Geometry check sheet. Reference: the model listing, model coordinates, mm. Face numbers are marked on the shaded views. A direction names the side the tool comes from. Round coordinates to 2 decimals unless told otherwise and drop trailing zeros. Loops run counter-clockwise (first coordinate to the right, second up) from the corner with the lowest first, then second, coordinate; pieces in that order, holes last. Notation, with made-up numbers: (-15.75, 78.25) -> (41.25, 78.25) arc R31 ccw to (41.25, 114.25) -> close; hole circle Ø5 at (-16.5, -30.5). An arc over 180 degrees is marked (long way). Use a Markdown table: item, result. Add a question column.
Q1. Gauge pin test, flat ends, axial feed: P1, Ø6.5, axis at x = -5, z = -3.5, coming from the +Y side; P2, Ø3, axis at x = 0.5, y = 4.5, coming from the -Z side; P3, Ø3, axis at x = -5.68, z = -3.75, coming from the +Y side; P4, Ø5.5, axis at x = 2.15, z = -3.75, coming from the +Y side. Record the tip position at first contact, or that the pin passes through.
Q2. Release check for a two-part mould opening along Z. For the marked faces 1, 2 and 3 record: released by +Z, released by -Z, zero draft, split by the parting line, or undercut.
Q3. Sectioned sample at B-B, the plane z = -6.5. Enter the section's corners in (x, y), then the cut area to 3 significant figures.
Q4. Sectioned sample at C-C, the plane x = -9.5. Enter the section's corners in (y, z), then the cut area to 3 significant figures.
Q5. Sectioned sample at D-D, the plane y = 2.5. Enter the section's corners in (x, z), then the cut area to 3 significant figures.
Q6. Set-up check for the marked faces 4, 5 and 6: record each of +Z, -Z, +X, -X, +Y, -Y from which the full face is reachable in a straight line by a thin tool's end or side.
Q7. Sectioned sample at A-A, the plane x = 2.5. Enter the section's corners in (y, z).
Q8. Material ranges on L1, parallel to Y at x = 2.5, z = 3.75; L2, parallel to X at y = 0.75, z = -3.25; L3, parallel to Z at x = -9, y = 1.5, recorded low to high.
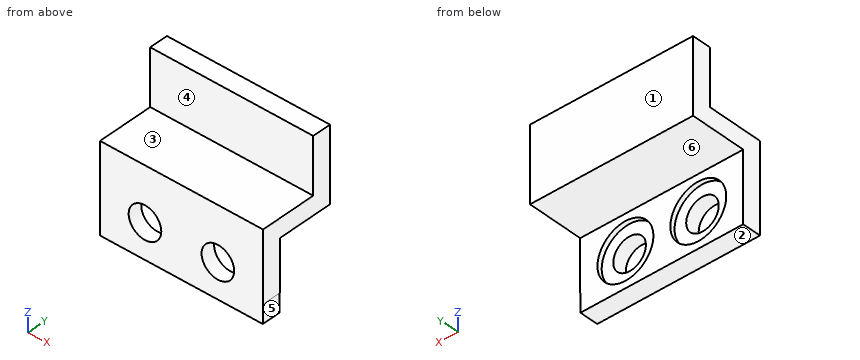
Autodesk Inventor part; units mm, degrees
ref_plane "YZ Plane" through (0, 0, 0) normal (1, 0, 0) x (0, 1, 0)
ref_plane "XZ Plane" through (0, 0, 0) normal (0, 1, 0) x (-1, 0, 0)
ref_plane "XY Plane" through (0, 0, 0) normal (0, 0, 1) x (1, 0, 0)
sketch "Boceto1" plane through (0, 0, 0) normal (0, 1, 0) x (-1, 0, 0)
  line L0 (0, 0) -> (3.5, 0)
  line L1 (3.5, 0) -> (5.5, 0)
  line L2 (0, 0) -> (-2, 0)
  line L3 (-2, -5.5) -> (5.5, -5.5)
  line L4 (-2, 0) -> (-5, 0)
  line L5 (-5, -5.5) -> (-2, -5.5)
  line L6 (5.5, 0) -> (8.5, 0)
  line L7 (8.5, -5.5) -> (5.5, -5.5)
  line L8 (8.5, -5.5) -> (9.5, -5.5)
  line L9 (9.5, 0) -> (8.5, 0)
  line L10 (-5, -5.5) -> (-6, -5.5)
  line L11 (-6, 0) -> (-5, 0)
  line L12 (9.5, -5.5) -> (10.5, -5.5)
  line L13 (10.5, -5.5) -> (10.5, 0)
  line L14 (10.5, 0) -> (9.5, 0)
  line L15 (-6, -5.5) -> (-7, -5.5)
  line L16 (-7, -5.5) -> (-7, 0)
  line L17 (-7, 0) -> (-6, 0)
  dimension "d30" = 1
  dimension "d37" = 1
  dimension "d38" = 1
extrude "Extrusión3" add sketch "Boceto1" along normal blind 2
sketch "Boceto4" plane through (-8.5, 0, 0) normal (0, 0, 1) x (1, 0, 0)
  line L0 (15.5, 2) -> (-2, 2)
  line L1 (0, 2) -> (13.5, 2)
  line L2 (13.5, 2) -> (13.5, 0)
  line L3 (13.5, 0) -> (0, 0)
  line L4 (0, 0) -> (0, 2)
  point P0 (8.5, 0)
  point P1 (14.5, 2)
  point P2 (-1, 2)
extrude "Extrusión4" add sketch "Boceto4" along normal blind 2
sketch "Boceto5" plane through (0, 2, 0) normal (0, 1, 0) x (1, 0, 0)
  line L0 (-8.5, -2) -> (5, -2)
  line L1 (5, -2) -> (-8.5, -2)
  line L2 (-8.5, -2) -> (-8.5, 0)
  line L3 (-8.5, 0) -> (5, 0)
  line L4 (5, 0) -> (5, -2)
  point P0 (0, 0)
extrude "Extrusión5" add sketch "Boceto5" along normal blind 6
sketch "Boceto6" plane through (-8.5, 0, 2) normal (0, 0, 1) x (1, 0, 0)
  line L0 (0, 0) -> (13.5, 0)
  line L1 (13.5, 0) -> (13.5, 6)
  line L2 (13.5, 6) -> (0, 6)
  line L3 (0, 0) -> (0, 6)
  line L4 (0, 0) -> (13.5, 0)
  line L5 (0, 0) -> (0, 8)
  line L6 (0, 8) -> (13.5, 8)
  line L7 (13.5, 8) -> (13.5, 6)
  line L8 (13.5, 6) -> (0, 6)
  line L9 (0, 6) -> (0, 8)
  point P0 (8.5, 0)
extrude "Extrusión6" add sketch "Boceto6" along normal blind 5 contours L5 L6 L7 L2
sketch "Boceto8" plane through (5, 0, -5.5) normal (0, 0, -1) x (-1, 0, 0)
  line L0 (13.5, 0) -> (13.5, 6)
  line L1 (13.5, 2) -> (0, 2)
  line L2 (13.5, 0) -> (0, 0)
  line L3 (0, 0) -> (0, 2)
  line L4 (0, 2) -> (13.5, 2)
  line L5 (13.5, 2) -> (13.5, 0)
  point P0 (5, 0)
extrude "Extrusión8" add sketch "Boceto8" along normal blind 2
sketch "Boceto11" plane through (5, 0, 2) normal (1, 0, 0) x (0, 0, -1)
  line L0 (-5, 8) -> (2, 8)
  line L1 (2, 8) -> (2, 6)
  line L2 (-5, 6) -> (-5, 8)
  line L3 (0, 0) -> (0, 6)
  line L4 (2, 0) -> (2, 2)
  line L5 (2, 6) -> (2, 0)
  line L6 (2, 0) -> (0, 0)
  line L7 (0, 0) -> (0, 6)
  line L8 (0, 6) -> (-5, 6)
  line L9 (0, 6) -> (-5, 6)
  line L10 (2, 0) -> (0, 0)
  line L11 (0, 0) -> (2, 0)
  line L12 (2, 2) -> (2, 8)
  line L13 (2, 0) -> (2, 8)
  line L14 (2, 8) -> (-5, 8)
  line L15 (2, 8) -> (-5, 8)
  line L16 (-5, 8) -> (-5, 6)
  line L17 (0, 6) -> (0, 0)
extrude "Extrusión11" add sketch "Boceto11" along normal blind 2
sketch "Boceto12" plane through (-8.5, 0, 0) normal (-1, 0, 0) x (0, 0, 1)
  line L0 (0, 8) -> (7, 8)
  line L1 (7, 8) -> (7, 6)
  line L2 (2, 6) -> (7, 6)
  line L3 (7, 6) -> (2, 6)
  line L4 (2, 6) -> (2, 0)
  line L5 (0, 0) -> (2, 0)
  line L6 (2, 0) -> (0, 0)
  line L7 (0, 2) -> (0, 8)
  line L8 (0, 0) -> (0, 8)
  line L9 (0, 8) -> (7, 8)
extrude "Extrusión12" add sketch "Boceto12" along normal blind 2
sketch "Boceto13" plane through (0, 2, 0) normal (0, 1, 0) x (1, 0, 0)
  line L0 (-8.5, 5.5) -> (-10.5, 5.5)
  line L1 (-10.5, 5.5) -> (6.9708, 5.5)
  line L2 (6.9708, 5.5) -> (6.9708, 7.5)
  line L3 (6.9708, 7.5) -> (-10.5, 7.5)
  line L4 (-10.5, 7.5) -> (-10.5, 5.5)
  point P0 (0, 0)
extrude "Extrusión13" add sketch "Boceto13" against normal blind 2
sketch "Boceto14" plane through (0, 2, 0) normal (0, 1, 0) x (1, 0, 0)
  circle A0 centre (2.1471, 3.7519) radius 1.75
  circle A1 centre (-5.6769, 3.7519) radius 1.75
  line L0 (1.1471, 3.7519) -> (2.1471, 3.7519)
  line L1 (-4.6769, 3.7519) -> (-5.6769, 3.7519)
  point P0 (0, 0)
  dimension "d43" = 3.5
  dimension "d44" = 3.5
  dimension "d45" = 1
  dimension "d46" = 1
extrude "Extrusión14" cut sketch "Boceto14" against normal blind 2
sketch "Boceto15" plane through (0, 2, 0) normal (0, 1, 0) x (1, 0, 0)
  circle A0 centre (2.1471, 3.7519) radius 1.75
  circle A1 centre (2.1471, 3.7519) radius 3
  circle A2 centre (-5.6769, 3.7519) radius 1.75
  circle A3 centre (-5.6769, 3.7519) radius 3
  point P0 (0, 0)
  dimension "d49" = 6
  dimension "d50" = 6
extrude "Extrusión15" cut sketch "Boceto15" against normal blind 0.5
sketch "Boceto16" plane through (-8.5, 0, 7) normal (0, 0, 1) x (1, 0, 0)
  line L0 (15.5, 2) -> (15.5, 8)
  line L1 (15.5, 6) -> (-2, 6)
  line L2 (15.5, 8) -> (-2, 8)
  line L3 (-2, 8) -> (-2, 6)
  line L4 (-2, 6) -> (15.5, 6)
  line L5 (15.5, 6) -> (15.5, 8)
  point P0 (8.5, 0)
extrude "Extrusión16" add sketch "Boceto16" along normal blind 1
properties part number "Pantalla - encaix slider"
Values:
| question | item | result |
|---|---|---|
| 1 | P1 | y = 2 |
| 1 | P2 | z = 0 |
| 1 | P3 | through |
| 1 | P4 | y = 1.5 |
| 2 | face 1 | zero draft |
| 2 | face 2 | released by -Z |
| 2 | face 3 | released by +Z |
| 3 | outline | (-10.5, 0) -> (6.97, 0) -> (6.97, 2) -> (3.35, 2) -> (3.35, 1.5) -> (0.94, 1.5) -> (0.94, 2) -> (-4.47, 2) -> (-4.47, 1.5) -> (-6.88, 1.5) -> (-6.88, 2) -> (-10.5, 2) -> close |
| 3 | area | 32.5 mm^2 |
| 4 | outline | (0, -7.5) -> (2, -7.5) -> (2, 0) -> (8, 0) -> (8, 8) -> (6, 8) -> (6, 2) -> (0, 2) -> close |
| 4 | area | 43.0 mm^2 |
| 5 | outline | (-10.5, 0) -> (7, 0) -> (7, 2) -> (-10.5, 2) -> close |
| 5 | area | 35.0 mm^2 |
| 6 | face 4 | +Z, +X, -X, -Y |
| 6 | face 5 | -Z, +X, +Y, -Y |
| 6 | face 6 | -Z, +X, -X, +Y |
| 7 | outline | (0, -7.5) -> (2, -7.5) -> (2, -6.73) -> (1.5, -6.73) -> (1.5, -5.47) -> (0, -5.47) -> close; (0, -2.04) -> (1.5, -2.04) -> (1.5, -0.77) -> (2, -0.77) -> (2, 0) -> (8, 0) -> (8, 8) -> (6, 8) -> (6, 2) -> (0, 2) -> close |
| 8 | L1 | 6 to 8 |
| 8 | L2 | -10.5 to -7.35, -4 to 0.47, 3.82 to 7 |
| 8 | L3 | -7.5 to 2 |
